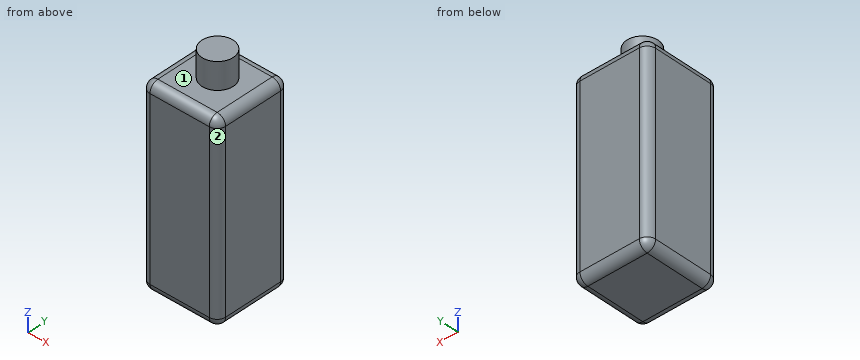
```python
from build123d import *

# Parameters (mm, degrees)
F0_W     = 44.955451
F0_H     = 112.923815
F1_DEPTH = 44.8
F2_R     = 5
F3_R     = 9.195935
F4_DEPTH = 15.6


with BuildPart() as f1:
    # F0 (on Front) → F1 (new body)
    with BuildSketch(Plane.XZ):
        with Locations((0.468286, -0.200692)):
            Rectangle(F0_W, F0_H)
    extrude(amount=F1_DEPTH)

    # F2
    f2_edges = [f1.edges().sort_by_distance(p)[0] for p in [
        (22.946011, -22.4, 56.261215),
        (0.468286, 0, 56.261215),
        (-22.00944, -22.4, 56.261215),
        (0.468286, -44.8, 56.261215),
        (22.946011, -22.4, -56.6626),
        (22.946011, -44.8, -0.200693),
        (22.946011, 0, -0.200693),
        (-22.00944, 0, -0.200693),
        (0.468286, 0, -56.6626),
        (-22.00944, -44.8, -0.200693),
        (-22.00944, -22.4, -56.6626),
        (0.468286, -44.8, -56.6626),
    ]]
    fillet(f2_edges, radius=F2_R)

    # F3 (on face) → F4 (join)
    with BuildSketch(Plane.XY.offset(56.261215)):
        with Locations((1.114632, -21.473374)):
            Circle(F3_R)
    extrude(amount=F4_DEPTH)


solid = f1.part
```
Design review of the part built by this model. Coordinates are the model's own, in mm. Face numbers are marked on the shaded views. A direction names the side the tool comes from. Round coordinates to 2 decimals unless told otherwise and drop trailing zeros. Order: outer loops, then holes, each group sorted by start corner. A loop starts at its lowest first (then second) coordinate and runs counter-clockwise, first axis right, second up. Notation, with made-up numbers: M 53,-6 L 107,-6 A30 ccw 107,29 Z; hole C -26.5,9.25 d3. An arc over 180 degrees is marked long. Put each result on its own line as item: value.
Q1. Consider section A-A (x = -14). State the section outline as (y, z) points, and give its area (3 significant figures).
Reported:
outline: M -44.8,-51.66 A5 ccw -39.8,-56.66 L -5,-56.66 A5 ccw 0,-51.66 L 0,51.26 A5 ccw -5,56.26 L -39.8,56.26 A5 ccw -44.8,51.26 Z
area: 5,040 mm²
Q2. Consider section C-C (z = 63). State the section outline as (x, y) points.
Reported:
outline: C 1.11,-21.47 d18.39
Q3. To check wall thickness, follow line 1 (Z direction, x = -10, y = -19.5); line 2 (Z direction, x = -17.5, y = -29); line 3 (X direction, y = -40, z = 45.5). State the ranges of each line that lie inside material, in increasing order.
Reported:
line 1: -56.66 to 56.26
line 2: -56.64 to 56.24
line 3: -22.01 to 22.94
Q4. Consider section D-D (y = -14). State the section outline as (x, z) points.
Reported:
outline: M -22.01,-51.66 A5 ccw -17.01,-56.66 L 17.95,-56.66 A5 ccw 22.95,-51.66 L 22.95,51.26 A5 ccw 17.95,56.26 L 6.47,56.26 L 6.47,71.86 L -4.24,71.86 L -4.24,56.26 L -17.01,56.26 A5 ccw -22.01,51.26 Z
Q5. Machinability: for the marked faces 1 and 2, which of the approach directions +Z, -Z, +X, -X, +Y, -Y give a long, thin tool a straight path to every point of the face, cutting with its end or side? Answer none if there is none.
Reported:
face 1: +Z
face 2: +Z, -Z, +X, -Y
Q6. Consider section B-B (y = -36.5). State the section outline as (x, z) points.
Reported:
outline: M -22.01,-51.66 A5 ccw -17.01,-56.66 L 17.95,-56.66 A5 ccw 22.95,-51.66 L 22.95,51.26 A5 ccw 17.95,56.26 L -17.01,56.26 A5 ccw -22.01,51.26 Z
Q7. Insertion check: pin 1 Ø1.5 at (x, y) = (-14.5, -36.5) entering from +Z; pin 2 Ø8 at (y, z) = (-21, 55.5) entering from -X. Each pin has a flat end and moves straight along its axis. Give the tip position at first contact, or say it passes through.
Reported:
pin 1: z = 56.26
pin 2: x = -22
